Work out the finished part from the listing and answer in its coordinate system (mm). A direction names the side the tool comes from. Coordinates: 2 decimals unless noted, no trailing zeros. Write each loop counter-clockwise with the first axis right and the second up, starting at its lowest first coordinate (ties: lowest second). Pieces come first, ordered by that corner, then holes. Notation, with made-up numbers: (55, -6.75) -> (103, -6.75) arc R31 cw to (103, 30.25) -> close; hole circle Ø10 at (21, 68.5). An arc over 180 degrees is marked (long way). Write each question's results on one line, items separated by ' | '. Start each with the question number.
from build123d import *

# Parameters (mm, degrees)
SKETCH_1_W          = 200
SKETCH_1_H          = 150
EXTRUDE_1_DEPTH     = 30
CUT_EXTRUDE_7_DEPTH = 12.5
CUT_EXTRUDE_8_DEPTH = 252.79356624
SKETCH_6_W          = 20
SKETCH_6_H          = 150
EXTRUDE_2_DEPTH     = 70
EXTRUDE_START       = -85
EXTRUDE_4_DEPTH     = 20
CUT_EXTRUDE_9_DEPTH = 20


with BuildPart() as part:
    # Эскиз1 → Бобышка-Вытянуть1 (new body)
    with BuildSketch(Plane.XY):
        with Locations((100, -75)):
            Rectangle(SKETCH_1_W, SKETCH_1_H)
    extrude(amount=EXTRUDE_1_DEPTH)

    # Эскиз2 → Вырез-Вытянуть7 (cut)
    with BuildSketch(Plane.XY.offset(30)):
        with BuildLine():
            Line((200, -105), (170, -105))
            ThreePointArc((170, -105), (160, -115), (170, -125))
            Line((170, -125), (200, -125))
            Line((200, -125), (200, -105))
        make_face()
        with BuildLine():
            Line((200, -25), (170, -25))
            ThreePointArc((170, -25), (160, -35), (170, -45))
            Line((170, -45), (200, -45))
            Line((200, -45), (200, -25))
        make_face()
    extrude(amount=-CUT_EXTRUDE_7_DEPTH, mode=Mode.SUBTRACT)

    # Эскиз5 → Вырез-Вытянуть8 (cut, through all)
    with BuildSketch(Plane.XY.offset(30)):
        with BuildLine():
            Line((0, -60), (20, -60))
            ThreePointArc((20, -60), (35, -75), (20, -90))
            Line((20, -90), (0, -90))
            Line((0, -90), (0, -60))
        make_face()
    extrude(amount=-CUT_EXTRUDE_8_DEPTH, mode=Mode.SUBTRACT)

    # Эскиз6 → Бобышка-Вытянуть2 (add)
    with BuildSketch(Plane.XY.offset(30)):
        with Locations((102.5, -75)):
            Rectangle(SKETCH_6_W, SKETCH_6_H)
    extrude(amount=EXTRUDE_2_DEPTH)

    # Эскиз7 → Бобышка-Вытянуть4 (add)
    with BuildSketch(Plane.XZ.offset(150).offset(EXTRUDE_START)):
        Polygon((112.5, 100), (200, 30), (112.5, 30), align=None)
    extrude(amount=EXTRUDE_4_DEPTH)

    # Эскиз10 → Вырез-Вытянуть9 (cut)
    with BuildSketch(Plane(origin=(112.5, 0, 0), x_dir=(0, 0, -1), z_dir=(1, 0, 0))):
        with BuildLine():
            Line((-52.5, -127.5), (-77.5, -127.5))
            ThreePointArc((-77.5, -127.5), (-87.5, -117.5), (-77.5, -107.5))
            Line((-77.5, -107.5), (-52.5, -107.5))
            ThreePointArc((-52.5, -107.5), (-42.5, -117.5), (-52.5, -127.5))
        make_face()
        with BuildLine():
            Line((-52.5, -22.5), (-77.5, -22.5))
            ThreePointArc((-77.5, -22.5), (-87.5, -32.5), (-77.5, -42.5))
            Line((-77.5, -42.5), (-52.5, -42.5))
            ThreePointArc((-52.5, -42.5), (-42.5, -32.5), (-52.5, -22.5))
        make_face()
    extrude(amount=-CUT_EXTRUDE_9_DEPTH, mode=Mode.SUBTRACT)


solid = part.part
1. Find the intervals of material crossed by L1, parallel to Y at x = 8, z = 16; L2, parallel to X at y = -38.5, z = 96.5; L3, parallel to Z at x = 118.5, y = -14, in increasing order.
2. Given pin 1 Ø1.5 at (x, z) = (128, 77) entering from +Y; pin 2 Ø21 at (y, z) = (-80.5, 59.5) entering from -X; pin 3 Ø8 at (x, y) = (50.5, -107.5) entering from +Z, each flat-ended and moving along its own axis, determine where each tip first touches the part or whether it passes through.
3. Find section B-B on x = 98.5. Give the vertices of the cut face in (y, z), and give its area (3 significant figures).
4. Find section C-C on y = -32.5. Give the vertices of the cut face in (x, z), and give its area (3 significant figures).
5. Find section A-A on z = 63. Give the vertices of the cut face in (x, y).
6. For faces 1 (the face through (156, -117, 30)), 2 (the face through (180, -115, 17.5)), 3 (the face through (103, -22.5, 65)), 4 (the face through (10, -60, 15)), 5 (the face through (156, -32, 30)), determine the directions among +Z, -Z, +X, -X, +Y, -Y from which every point of the face is accessible in a straight line to the end or side of a thin tool.
7. Find section D-D on x = 183. Give the vertices of the cut face in (y, z).
8. Determine the mould class of faces 6 (the face through (46, -74, 30)), 7 (the face through (103, -107.5, 65)), 8 (the face through (92.5, -76, 65)) for opening direction Z: pulls with the +Z half, pulls with the -Z half, needs draft (parallel to the pull), parting line crosses it, or undercut.
Ans:
1) L1: y = -150 to -90, -60 to 0 | L2: x = 92.5 to 112.5 | L3: z = 0 to 30
2) pin 1: stops at y = -65 | pin 2: stops at x = 92.5 | pin 3: stops at z = 30
3) outline: (-150, 0) -> (0, 0) -> (0, 100) -> (-150, 100) -> close; hole (-127.5, 52.5) arc R10 ccw to (-107.5, 52.5) -> (-107.5, 77.5) arc R10 ccw to (-127.5, 77.5) -> close; hole (-42.5, 52.5) arc R10 ccw to (-22.5, 52.5) -> (-22.5, 77.5) arc R10 ccw to (-42.5, 77.5) -> close | area: 13,400 mm²
4) outline: (0, 0) -> (200, 0) -> (200, 17.5) -> (160.32, 17.5) -> (160.32, 30) -> (112.5, 30) -> (112.5, 42.5) -> (92.5, 42.5) -> (92.5, 30) -> (0, 30) -> close; (92.5, 87.5) -> (112.5, 87.5) -> (112.5, 100) -> (92.5, 100) -> close | area: 6,000 mm²
5) outline: (92.5, -150) -> (112.5, -150) -> (112.5, -127.5) -> (92.5, -127.5) -> close; (92.5, -107.5) -> (112.5, -107.5) -> (112.5, -85) -> (158.75, -85) -> (158.75, -65) -> (112.5, -65) -> (112.5, -42.5) -> (92.5, -42.5) -> close; (92.5, -22.5) -> (112.5, -22.5) -> (112.5, 0) -> (92.5, 0) -> close
6) face 1: +Z, +X, -Y | face 2: +Z, +X | face 3: +X, -X | face 4: +Z, -Z, -X | face 5: +Z, +X, +Y
7) outline: (-150, 0) -> (0, 0) -> (0, 30) -> (-25, 30) -> (-25, 17.5) -> (-45, 17.5) -> (-45, 30) -> (-65, 30) -> (-65, 43.6) -> (-85, 43.6) -> (-85, 30) -> (-105, 30) -> (-105, 17.5) -> (-125, 17.5) -> (-125, 30) -> (-150, 30) -> close
8) face 6: pulls with the +Z half | face 7: undercut | face 8: needs draft
